For this review, take the finished solid that the model builds, in its own axes (mm). Face numbers are marked on the shaded views. A direction names the side the tool comes from. Coordinates: 2 decimals unless noted, no trailing zeros. Loops run counter-clockwise (first coordinate to the right, second up) from the corner with the lowest first, then second, coordinate; pieces in that order, holes last. Notation, with made-up numbers: (41, 9) -> (77, 9) arc R15 cw to (77, 23) -> close; hole circle Ø4 at (8, 11). An arc over 180 degrees is marked (long way). One line per item, written item: value.
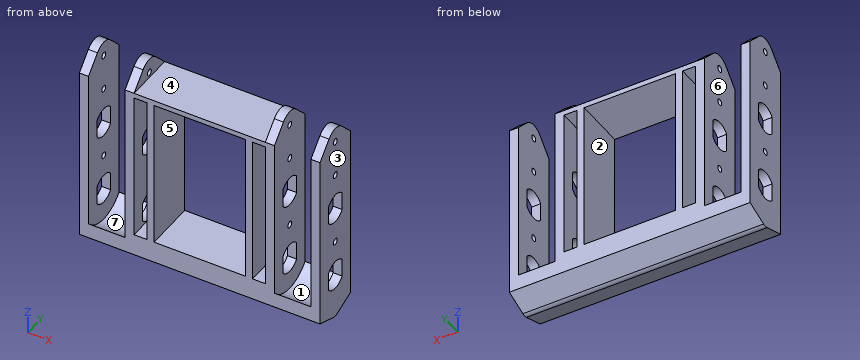
from build123d import *

# Parameters (mm, degrees)
BOSS_EXTRUDE1_DEPTH = 66
CUT_EXTRUDE3_START  = -5
CUT_EXTRUDE3_DEPTH  = 20
CUT_EXTRUDE4_START  = -5
SKETCH5_W           = 82.2
SKETCH5_H           = 28
CUT_EXTRUDE4_DEPTH  = 7
CUT_EXTRUDE5_START  = 29
SKETCH1_13_R        = 1.75
CUT_EXTRUDE5_DEPTH  = 37
SKETCH7_W           = 72
SKETCH7_H           = 11
CUT_EXTRUDE7_DEPTH  = 97.605188784
SKETCH8_W           = 50
SKETCH8_H           = 82.2
CUT_EXTRUDE8_DEPTH  = 97.605188784


with BuildPart() as part:
    # Sketch1 → Boss-Extrude1 (new, symmetric)
    with BuildSketch(Plane(origin=(0, 0, 0), x_dir=(0, 0, -1), z_dir=(1, 0, 0))):
        with BuildLine():
            Line((60, 14), (64.468246011, 1.611607143))
            ThreePointArc((64.468246011, 1.611607143), (64.75, 0), (64.468246011, -1.611607143))
            Line((64.468246011, -1.611607143), (60, -14))
            Line((60, -14), (-37, -14))
            Line((-37, -14), (-45.550860067, -5.760898586))
            ThreePointArc((-45.550860067, -5.760898586), (-48, 0), (-45.550860067, 5.760898586))
            Line((-45.550860067, 5.760898586), (-37, 14))
            Line((-37, 14), (60, 14))
        make_face()
    extrude(amount=BOSS_EXTRUDE1_DEPTH, both=True)

    # Sketch4 → Cut-Extrude3 (cut)
    with BuildSketch(Plane(origin=(66, 0, 0), x_dir=(0, 0, -1), z_dir=(1, 0, 0)).offset(CUT_EXTRUDE3_START)):
        with BuildLine():
            ThreePointArc((51.707369474, -14), (58.25, 0), (51.707369474, 14))
            Line((51.707369474, 14), (-37, 14))
            Line((-37, 14), (-45.550860067, 5.760898586))
            ThreePointArc((-45.550860067, 5.760898586), (-48, 0), (-45.550860067, -5.760898586))
            Line((-45.550860067, -5.760898586), (-37, -14))
            Line((-37, -14), (51.707369474, -14))
        make_face()
    cut_extrude3 = extrude(amount=-CUT_EXTRUDE3_DEPTH, mode=Mode.SUBTRACT)

    # Sketch5 → Cut-Extrude4 (cut)
    with BuildSketch(Plane(origin=(41, 0, 0), x_dir=(0, 0, -1), z_dir=(1, 0, 0)).offset(CUT_EXTRUDE4_START)):
        with Locations((6.9, 0)):
            Rectangle(SKETCH5_W, SKETCH5_H)
    cut_extrude4 = extrude(amount=-CUT_EXTRUDE4_DEPTH, mode=Mode.SUBTRACT)

    # Sketch1<13> → Cut-Extrude5 (cut)
    with BuildSketch(Plane(origin=(0, 0, 0), x_dir=(0, 0, -1), z_dir=(1, 0, 0)).offset(CUT_EXTRUDE5_START)):
        with BuildLine():
            Line((4.993746089, -6.25), (-4.993746089, -6.25))
            ThreePointArc((-4.993746089, -6.25), (-8, 0), (-4.993746089, 6.25))
            Line((-4.993746089, 6.25), (4.993746089, 6.25))
            ThreePointArc((4.993746089, 6.25), (8, 0), (4.993746089, -6.25))
        make_face()
        with BuildLine():
            Line((44.993746089, -6.25), (35.006253911, -6.25))
            ThreePointArc((35.006253911, -6.25), (32, 0), (35.006253911, 6.25))
            Line((35.006253911, 6.25), (44.993746089, 6.25))
            ThreePointArc((44.993746089, 6.25), (48, 0), (44.993746089, -6.25))
        make_face()
        with Locations((-20, 0)):
            Circle(SKETCH1_13_R)
        with Locations((20, 0)):
            Circle(SKETCH1_13_R)
        with Locations((-40, 0)):
            Circle(SKETCH1_13_R)
    cut_extrude5 = extrude(amount=CUT_EXTRUDE5_DEPTH, mode=Mode.SUBTRACT)

    # Mirror2: Cut-Extrude3, Cut-Extrude4, Cut-Extrude5 across plane
    add(cut_extrude3.mirror(Plane(origin=(0, 0, 0), x_dir=(0, 0, 1), z_dir=(1, 0, 0))), mode=Mode.SUBTRACT)
    add(cut_extrude4.mirror(Plane(origin=(0, 0, 0), x_dir=(0, 0, 1), z_dir=(1, 0, 0))), mode=Mode.SUBTRACT)
    add(cut_extrude5.mirror(Plane(origin=(0, 0, 0), x_dir=(0, 0, 1), z_dir=(1, 0, 0))), mode=Mode.SUBTRACT)

    # Sketch7 → Cut-Extrude7 (cut, through all)
    with BuildSketch(Plane(origin=(0, 14, 0), x_dir=(1, 0, 0), z_dir=(0, 1, 0))):
        with Locations((0, -42.5)):
            Rectangle(SKETCH7_W, SKETCH7_H)
    extrude(amount=-CUT_EXTRUDE7_DEPTH, mode=Mode.SUBTRACT)

    # Sketch8 → Cut-Extrude8 (cut, through all)
    with BuildSketch(Plane(origin=(0, 14, 0), x_dir=(1, 0, 0), z_dir=(0, 1, 0))):
        with Locations((0, 6.9)):
            Rectangle(SKETCH8_W, SKETCH8_H)
    extrude(amount=-CUT_EXTRUDE8_DEPTH, mode=Mode.SUBTRACT)


solid = part.part
1. The part is to be moulded in two halves that separate along Z. For the marked faces 5, 6 and 7, say which applies: pulls with the +Z half, pulls with the -Z half, needs draft (parallel to the pull), parting line crosses it, or undercut.
Return value:
face 5: undercut
face 6: needs draft
face 7: pulls with the +Z half
2. For the marked faces 1, 2, 3 and 4, list the 3-axis set-ups (+Z, -Z, +X, -X, +Y, -Y) from which the entire face can be reached by the end or side of a thin tool; tool diameter is ignored.
Return value:
face 1: +Z
face 2: +Y, -Y
face 3: +Z, -Z, +X, +Y, -Y
face 4: +Z, +Y, -Y
3. Insertion check: pin 1 Ø2 at (y, z) = (0, 20) entering from +X; pin 2 Ø1 at (x, y) = (-43.5, 5.5) entering from +Z; pin 3 Ø8 at (x, y) = (-3, -2.5) entering from +Z. Each pin has a flat end and moves straight along its axis. Give the tip position at first contact, or say it passes through.
Return value:
pin 1: stops at x = 29
pin 2: stops at z = -57.24
pin 3: stops at z = 37
4. Take a section at D-D, the plane z = 20. Give the number of separate pieces and of enclosed holes in the cut face, and give its area (3 significant figures).
Return value:
separate pieces: 10
enclosed holes: 0
area: 714 mm2
5. Take a section at A-A, the plane z = -23.5. Give the boundary of the cut face in (x, y), and give its area (3 significant figures).
Return value:
outline: (-66, -14) -> (-61, -14) -> (-61, 14) -> (-66, 14) -> close; (-41, -14) -> (-36, -14) -> (-36, 14) -> (-41, 14) -> close; (-29, -14) -> (-25, -14) -> (-25, 14) -> (-29, 14) -> close; (25, -14) -> (29, -14) -> (29, 14) -> (25, 14) -> close; (36, -14) -> (41, -14) -> (41, 14) -> (36, 14) -> close; (61, -14) -> (66, -14) -> (66, 14) -> (61, 14) -> close
area: 784 mm2
6. To check wall thickness, follow probe 1 along X at (y, z) = (-11.25, 7.5); probe 2 along X at (y, z) = (2.75, -36.5); probe 3 along Y at (x, z) = (-64, -20). State the ranges of each line that lie inside material, in increasing order. Write a range as from..to.
Return value:
probe 1: x = -66..-61, -41..-36, -29..-25, 25..29, 36..41, 61..66
probe 2: x = -29..-25, 25..29
probe 3: y = -14..-1.75, 1.75..14
7. Take a section at B-B, the plane x = 3. Give the boundary of the cut face in (y, z), and give its area (3 significant figures).
Return value:
outline: (-14, -60) -> (-1.61, -64.47) arc R4.75 ccw to (1.61, -64.47) -> (14, -60) -> (14, -48) -> (-14, -48) -> close; (-14, 34.2) -> (14, 34.2) -> (14, 37) -> (-14, 37) -> close
area: 485 mm2
8. Take a section at C-C, the plane y = -8. Give the boundary of the cut face in (x, z), and give its area (3 significant figures).
Return value:
outline: (-66, -62.16) -> (66, -62.16) -> (66, 43.23) -> (61, 43.23) -> (61, -56.4) -> (41, -56.4) -> (41, 43.23) -> (36, 43.23) -> (36, 37) -> (-36, 37) -> (-36, 43.23) -> (-41, 43.23) -> (-41, -56.4) -> (-61, -56.4) -> (-61, 43.23) -> (-66, 43.23) -> close; hole (-36, -48) -> (-29, -48) -> (-29, 34.2) -> (-36, 34.2) -> close; hole (-25, -48) -> (25, -48) -> (25, 34.2) -> (-25, 34.2) -> close; hole (29, -48) -> (36, -48) -> (36, 34.2) -> (29, 34.2) -> close
area: 4,220 mm2
